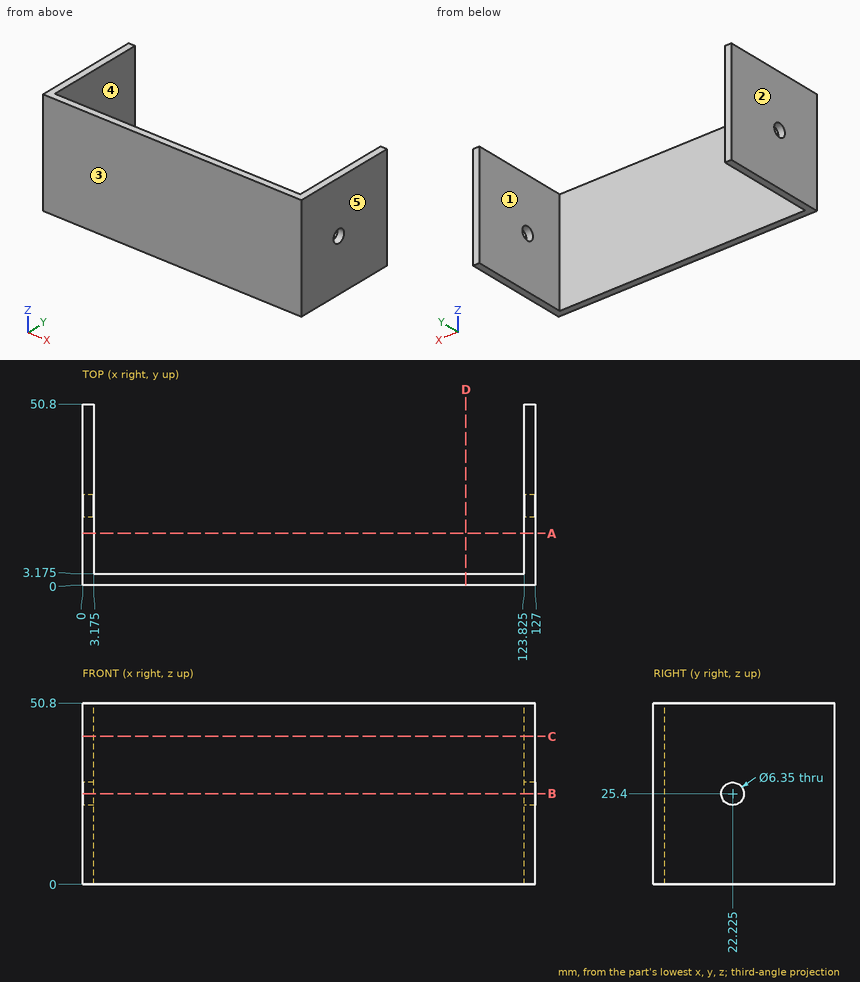
Can you work these out from the drawing? Everything is in mm from the part's minimum corner. A direction names the side the tool comes from. Give positions to 0.01 mm unless a question says otherwise; leave off trailing zeros. Loops run counter-clockwise (first coordinate to the right, second up) from the corner with the lowest first, then second, coordinate; pieces in that order, holes last. Notation, with made-up numbers: (29.25, 67.25) -> (78.25, 67.25) arc R33 ccw to (78.25, 102.25) -> close; hole circle Ø9 at (-26.5, 48.5). An arc over 180 degrees is marked (long way). Return JSON: item names as keys, results as strings.
Item 1: I need wall thicknesses on L1, parallel to Y at x = 1, z = 25; L2, parallel to X at y = 18, z = 45 (3 decimals); L3, parallel to Y at x = 44.5, z = 27.5 (3 decimals). Which ranges of each line are inside material? Lowest first, please. Write a range as from..to.
Geometry results:
{"L1": "y = 0..19.08, 25.37..50.8", "L2": "x = 0..3.175, 123.825..127", "L3": "y = 0..3.175"}
Item 2: If we section it at C-C on z = 41.5: List the corners of the cut face in (x, y) for me (3 decimals).
Geometry results:
{"outline": "(0, 0) -> (127, 0) -> (127, 50.8) -> (123.825, 50.8) -> (123.825, 3.175) -> (3.175, 3.175) -> (3.175, 50.8) -> (0, 50.8) -> close"}
Item 3: If we section it at D-D on x = 107.5: List the corners of the cut face in (y, z) for me (3 decimals), plus the area to 3 significant figures.
Geometry results:
{"outline": "(0, 0) -> (3.175, 0) -> (3.175, 50.8) -> (0, 50.8) -> close", "area": "161 mm²"}
Item 4: We'd pull the mould along X, two halves only. Please class the marked faces 1, 2 and 3: +X half, -X half, draft (parallel to the pull), parting line (faces both ways), or undercut.
Geometry results:
{"face 1": "undercut", "face 2": "-X half", "face 3": "draft"}
Item 5: If we section it at B-B on z = 25.4: List the corners of the cut face in (x, y) for me (3 decimals).
Geometry results:
{"outline": "(0, 0) -> (127, 0) -> (127, 19.05) -> (123.825, 19.05) -> (123.825, 3.175) -> (3.175, 3.175) -> (3.175, 19.05) -> (0, 19.05) -> close; (0, 25.4) -> (3.175, 25.4) -> (3.175, 50.8) -> (0, 50.8) -> close; (123.825, 25.4) -> (127, 25.4) -> (127, 50.8) -> (123.825, 50.8) -> close"}
Item 6: Which directions (+Z, -Z, +X, -X, +Y, -Y) give clear straight access to the entire face, cutting with the end or side of a thin tool? Please do the marked faces 4 and 5.
Geometry results:
{"face 4": "+Z, -Z, +Y", "face 5": "+Z, -Z, +X, +Y, -Y"}
Item 7: If we section it at A-A on y = 14.5: List the corners of the cut face in (x, z) for me (3 decimals).
Geometry results:
{"outline": "(0, 0) -> (3.175, 0) -> (3.175, 50.8) -> (0, 50.8) -> close; (123.825, 0) -> (127, 0) -> (127, 50.8) -> (123.825, 50.8) -> close"}
Item 8: I'm going to push a flat-ended pin straight in: pin 1 (12 mm diameter, centred on x = 68, z = 41.5, fed in from +Y) (3 decimals). Where does the tip first touch, or does it pass through?
Geometry results:
{"pin 1": "stops at y = 3.175"}
